Autodesk Inventor part; units mm, degrees
ref_plane "YZ Plane" through (0, 0, 0) normal (1, 0, 0) x (0, 1, 0)
ref_plane "XZ Plane" through (0, 0, 0) normal (0, 1, 0) x (-1, 0, 0)
ref_plane "XY Plane" through (0, 0, 0) normal (0, 0, 1) x (1, 0, 0)
sketch "Sketch1" plane through (0, 0, 0) normal (0, 1, 0) x (-1, 0, 0)
  line L0 (69.85, 9.525) -> (-69.85, 9.525)
  line L1 (-69.85, 9.525) -> (-69.85, -9.525)
  line L2 (-69.85, -9.525) -> (69.85, -9.525)
  line L3 (69.85, -9.525) -> (69.85, 9.525)
  line L4 (69.85, 9.525) -> (-69.85, -9.525) construction
  line L5 (-69.85, 9.525) -> (69.85, -9.525) construction
  point P0 (0, 0)
  dimension "d0" = 139.7
  dimension "d1" = 19.05
extrude "Extrusion1" add sketch "Sketch1" along normal blind 19.3675
sketch "Sketch2" plane through (-69.85, 0, 9.525) normal (0, 0, 1) x (1, 0, 0)
  line L0 (0, 19.3675) -> (139.7, 19.3675)
  arc A0 (55.245, 19.3675) -> (84.455, 19.3675) centre (69.85, 19.3675) ccw
  point P0 (69.85, 0)
  dimension "d4" = 29.21
extrude "Extrusion2" cut sketch "Sketch2" against normal through all
sketch "Sketch3" plane through (0, 19.3675, 0) normal (0, 1, 0) x (1, 0, 0)
  line L0 (-69.85, -9.525) -> (-14.605, -9.525)
  line L1 (-69.85, 9.525) -> (-69.85, -9.525)
  line L2 (-14.605, 9.525) -> (-69.85, 9.525)
  line L3 (69.85, -9.525) -> (69.85, 9.525)
  line L4 (69.85, 9.525) -> (14.605, 9.525)
  line L5 (14.605, -9.525) -> (69.85, -9.525)
  point P0 (0, 0)
  point P1 (-57.15, 0)
  point P2 (57.15, 0)
  dimension "d7" = 9.525
  dimension "d8" = 12.7
  dimension "d13" = 9.525
  dimension "d14" = 12.7
hole "Hole1" at (-57.15, 19.3675, 0) at (57.15, 19.3675, 0) direction (0, -1, 0) diameter 7.1374 end through all
properties part number "BaseOfSwallowWatererV01"
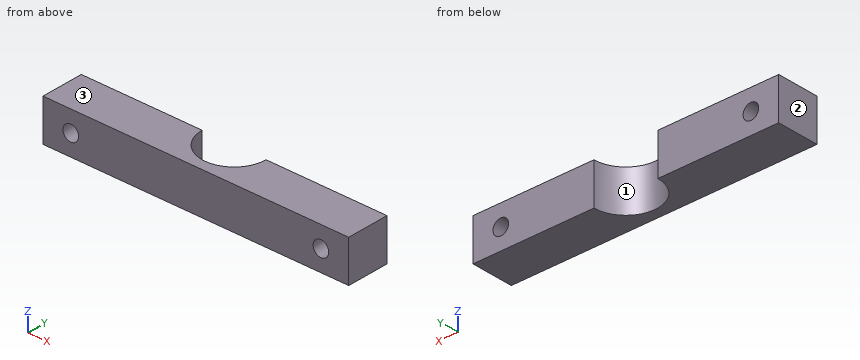
Verification items for the finished model (mm, model axes). Face numbers are marked on the shaded views. Coordinates: 2 decimals unless noted, no trailing zeros. Loops run counter-clockwise (first coordinate to the right, second up) from the corner with the lowest first, then second, coordinate; pieces in that order, holes last. Notation, with made-up numbers: (80, 56) - (120, 56) arc R35 cw to (120, 95) - close; hole circle Ø11 at (79, 73). An arc over 180 degrees is marked (long way). Answer as a JSON object with one key per item and string values.
(1) Cross-section at B-B, the plane z = 0. Count the separate pieces of the cut face and the enclosed holes in it, then the cut area to 3 significant figures.
Response:
{"separate pieces": "3", "enclosed holes": "0", "area": "2,090 mm²"}
(2) Cross-section at A-A, the plane x = -57.15. Record the boundary of the cut face in (y, z) (1 decimal).
Response:
{"outline": "(0, -9.5) - (19.4, -9.5) - (19.4, -3.6) - (0, -3.6) - close; (0, 3.6) - (19.4, 3.6) - (19.4, 9.5) - (0, 9.5) - close"}
(3) Mould release check, pull along X, two halves, no side actions. Record for the marked faces 1, 2 and 3: pulls with the +X half, pulls with the -X half, needs draft (parallel to the pull), parting line crosses it, or undercut.
Response:
{"face 1": "undercut", "face 2": "pulls with the -X half", "face 3": "needs draft"}
(4) Go/stop test with flat-tipped pins: pin 1 Ø4.5 at (x, z) = (-57.15, 0) entering from -Y; pin 2 Ø2 at (x, z) = (4, -3) entering from +Y. Record where each tip stops, or that it passes through.
Response:
{"pin 1": "passes through", "pin 2": "stops at y = 5.65"}
(5) Cross-section at C-C, the plane y = 8.5. Record the boundary of the cut face in (x, z) (3 decimals), then the cut area to 3 significant figures.
Response:
{"outline": "(-69.85, -9.525) - (-9.757, -9.525) - (-9.757, 9.525) - (-69.85, 9.525) - close; (9.757, -9.525) - (69.85, -9.525) - (69.85, 9.525) - (9.757, 9.525) - close; hole circle Ø7.137 at (-57.15, 0); hole circle Ø7.137 at (57.15, 0)", "area": "2,210 mm²"}
(6) Scan lines: line 1 along X through (y, z) = (4.5, 0); line 2 along X through (y, z) = (14.75, 0); line 3 along Z through (x, y) = (57.15, 13.5) (3 decimals). Record each from-to range of solid material in increasing order.
Response:
{"line 1": "x = -69.85 to -60.72, -53.58 to 53.58, 60.72 to 69.85", "line 2": "x = -69.85 to -60.72, -53.58 to -13.86, 13.86 to 53.58, 60.72 to 69.85", "line 3": "z = -9.525 to -3.569, 3.569 to 9.525"}
